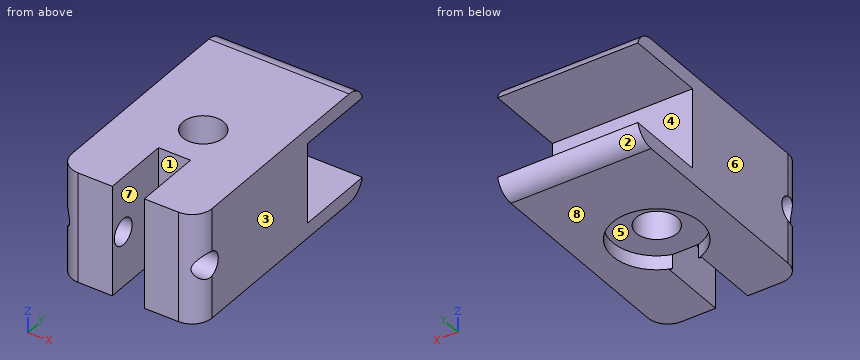
from build123d import *

# Parameters (mm, degrees)
CROQUIS1_W              = 35
CROQUIS1_H              = 35
CROQUIS1_R              = 11
ENTRADABASE_DEPTH       = 3.5
CROQUIS2_W              = 35
CROQUIS2_H              = 35
CROQUIS2_R              = 5.1
ENTRADACAVIDAD_DEPTH    = 24
REDONDEO1_R             = 5
CROQUIS4_W              = 27.5
CROQUIS4_H              = 14.86
CROQUIS4_R              = 3.25
BARRENORODAMIENTO_DEPTH = 35
CROQUIS5_W              = 8
CROQUIS5_H              = 16.86
ENTRADARODAMIENTO_DEPTH = 64.195487181
DETALLE2_R              = 5
CROQUIS10_W             = 3.75
CROQUIS10_H             = 15
SALIENTE_EXTRUIR4_DEPTH = 35
REDONDEO5_R             = 5
CROQUIS11_W             = 20
CROQUIS11_H             = 20
CORTAR_EXTRUIR5_DEPTH   = 64.195487351


with BuildPart() as part:
    # Croquis1 → EntradaBase (new body)
    with BuildSketch(Plane.XY):
        with Locations((17.5, -17.5)):
            Rectangle(CROQUIS1_W, CROQUIS1_H)
        with Locations((17.5, -17.5)):
            Circle(CROQUIS1_R, mode=Mode.SUBTRACT)
    extrude(amount=ENTRADABASE_DEPTH)

    # Croquis2 → EntradaCavidad (add)
    with BuildSketch(Plane.XY.offset(3.5)):
        with Locations((17.5, -17.5)):
            Rectangle(CROQUIS2_W, CROQUIS2_H)
        with Locations((17.5, -17.5)):
            Circle(CROQUIS2_R, mode=Mode.SUBTRACT)
    extrude(amount=ENTRADACAVIDAD_DEPTH)

    # Redondeo1
    redondeo1_edges = [part.edges().sort_by_distance(p)[0] for p in [
        (35, -35, 13.75),
        (0, -35, 13.75),
    ]]
    fillet(redondeo1_edges, radius=REDONDEO1_R)

    # Croquis4 → BarrenoRodamiento (add, through all)
    with BuildSketch(Plane.ZY):
        with Locations((13.75, -37.43)):
            Rectangle(CROQUIS4_W, CROQUIS4_H)
        with Locations(Location((13.75, -40.86, 0), (0, 0, 270))):
            Circle(CROQUIS4_R, mode=Mode.SUBTRACT)
    extrude(amount=-BARRENORODAMIENTO_DEPTH)

    # Croquis5 → EntradaRodamiento (cut, through all)
    with BuildSketch(Plane(origin=(0, 0, 0), x_dir=(-1, 0, 0), z_dir=(0, 0, -1))):
        with Locations((-17.5, -36.43)):
            Rectangle(CROQUIS5_W, CROQUIS5_H)
    extrude(amount=-ENTRADARODAMIENTO_DEPTH, mode=Mode.SUBTRACT)

    # Detalle2
    # the kernel refuses this fillet: 5 mm, written as the material it takes off along each edge
    with BuildSketch(Plane(origin=(35, -44.86, -12.5), x_dir=(-1, 0, 0), z_dir=(0, 0, 1))) as detalle2_piece_1:
        with BuildLine():
            CenterArc((DETALLE2_R, -DETALLE2_R), DETALLE2_R, 90, 90)
            Line((0, -DETALLE2_R), (0, 0))
            Line((0, 0), (DETALLE2_R, 0))
        make_face()
    extrude(amount=52.5, mode=Mode.SUBTRACT)
    with BuildSketch(Plane(origin=(0, -44.86, -12.5), x_dir=(1, 0, 0), z_dir=(0, 0, 1))) as detalle2_piece_2:
        with BuildLine():
            CenterArc((DETALLE2_R, DETALLE2_R), DETALLE2_R, 180, 90)
            Line((0, DETALLE2_R), (0, 0))
            Line((0, 0), (DETALLE2_R, 0))
        make_face()
    extrude(amount=52.5, mode=Mode.SUBTRACT)

    # Croquis10 → Saliente-Extruir4 (add, through all)
    with BuildSketch(Plane.ZY):
        with Locations((1.875, 7.5)):
            Rectangle(CROQUIS10_W, CROQUIS10_H)
        with Locations((25.625, 7.5)):
            Rectangle(CROQUIS10_W, CROQUIS10_H)
    extrude(amount=-SALIENTE_EXTRUIR4_DEPTH)

    # Redondeo5
    # the kernel refuses this fillet: 5 mm, written as the material it takes off along each edge
    with BuildSketch(Plane(origin=(-12.103072957, 15, 0), x_dir=(0, -1, 0), z_dir=(1, 0, 0))) as redondeo5_piece_1:
        with BuildLine():
            CenterArc((4.841229183, -5), REDONDEO5_R, 90, 75.522487814)
            Line((0, -3.75), (-0.096824584, -3.725))
            ThreePointArc((-0.096824584, -3.725), (-0.1, -1.875), (-0.1, 0))
            Line((-0.1, 0), (0, 0.1))
            Line((0, 0.1), (4.841229183, 0.1))
            Line((4.841229183, 0.1), (4.841229183, 0))
        make_face()
    extrude(amount=59.206145914, mode=Mode.SUBTRACT)
    with BuildSketch(Plane(origin=(-12.103072957, 15, 27.5), x_dir=(0, -1, 0), z_dir=(1, 0, 0))) as redondeo5_piece_2:
        with BuildLine():
            CenterArc((4.841229183, 5), REDONDEO5_R, 194.477512186, 75.522487814)
            Line((0, 3.75), (-0.096824584, 3.725))
            ThreePointArc((-0.096824584, 3.725), (-0.1, 1.875), (-0.1, 0))
            Line((-0.1, 0), (0, -0.1))
            Line((0, -0.1), (4.841229183, -0.1))
            Line((4.841229183, -0.1), (4.841229183, 0))
        make_face()
    extrude(amount=59.206145914, mode=Mode.SUBTRACT)

    # Croquis11 → Cortar-Extruir5 (cut, through all)
    with BuildSketch(Plane.ZY):
        with Locations((13.75, 5)):
            Rectangle(CROQUIS11_W, CROQUIS11_H)
    extrude(amount=-CORTAR_EXTRUIR5_DEPTH, mode=Mode.SUBTRACT)


solid = part.part
The listing builds one solid part. Answer for the finished solid, in the listing's coordinates (mm). Face numbers are marked on the shaded views. A direction names the side the tool comes from. Round coordinates to 2 decimals unless told otherwise and drop trailing zeros. Write each loop counter-clockwise with the first axis right and the second up, starting at its lowest first coordinate (ties: lowest second). Pieces come first, ordered by that corner, then holes. Notation, with made-up numbers: (54, 78) - (88, 78) arc R11 cw to (88, 92) - close; hole circle Ø9 at (77.25, 45). An arc over 180 degrees is marked (long way). Use a Markdown table: item, result. Add a question column.
1. The part is cut by section B-B (y = -32). Write down the section's boundary in (x, z), and give its area (4 significant figures).
2. A tool of negligible diameter and unlimited length cuts with its end or side. For the marked faces 1, 2, 3, 4 and 5, from which of +Z, -Z, +X, -X, +Y, -Y can it reach the whole face along a straight path? Write none if from no direction.
3. The part is cut by section A-A (x = 17.5). Write down the section's boundary in (y, z).
4. Consider line 1 (X direction, y = -32, z = 19.5); line 2 (Z direction, x = 13.5, y = -4); line 3 (Y direction, x = 25.5, z = 13.75). Determine where each line is inside the solid, lowest interval first.
5. For a pull along X with two mould halves and no side action, classify the marked faces 6, 7 and 8 as +X half, -X half, draft (parallel to the pull), parting line (faces both ways), or undercut.
6. The part is cut by section C-C (z = 15.5). Write down the section's boundary in (x, y).
7. The part is cut by section D-D (z = 4.5). Write down the section's boundary in (x, y), and give its area (3 significant figures).
8. Flat-ended cylindrical pins translate along their axes: P1, Ø1, axis at x = 20, z = 20, coming from the -Y side; P2, Ø10, axis at x = 20.5, z = 16.5, coming from the +Y side. Find the tip coordinate at first contact, or state that the pin passes through.
Reported:
| question | item | result |
|---|---|---|
| 1 | outline | (0, 0) - (13.5, 0) - (13.5, 27.5) - (0, 27.5) - close; (21.5, 0) - (35, 0) - (35, 27.5) - (21.5, 27.5) - close |
| 1 | area | 742.5 mm^2 |
| 2 | face 1 | +Z, -Z, -Y |
| 2 | face 2 | -Z, +X, -X, +Y |
| 2 | face 3 | +Z, -Z, +X, +Y, -Y |
| 2 | face 4 | +X, -X, +Y |
| 2 | face 5 | -Z |
| 3 | outline | (-28, 3.5) - (-22.6, 3.5) - (-22.6, 27.5) - (-28, 27.5) - close; (-12.4, 3.5) - (-6.5, 3.5) - (-6.5, 0) - (10.16, 0) arc R5 ccw to (15, 3.75) - (-5, 3.75) - (-5, 23.75) - (15, 23.75) arc R5 ccw to (10.16, 27.5) - (-12.4, 27.5) - close |
| 4 | line 1 | 0 to 13.5, 21.5 to 35 |
| 4 | line 2 | 0 to 3.75, 23.75 to 27.5 |
| 4 | line 3 | -44.86 to -44.11, -37.61 to -5 |
| 5 | face 6 | -X half |
| 5 | face 7 | undercut |
| 5 | face 8 | draft |
| 6 | outline | (0, -38.12) - (13.5, -38.12) - (13.5, -28) - (21.5, -28) - (21.5, -38.12) - (35, -38.12) - (35, -5) - (0, -5) - close; (1.68, -43.6) arc R5 ccw to (5, -44.86) - (13.5, -44.86) - (13.5, -43.6) - close; (21.5, -44.86) - (30, -44.86) arc R5 ccw to (33.32, -43.6) - (21.5, -43.6) - close; hole circle Ø10.2 at (17.5, -17.5) |
| 7 | outline | (0, -39.86) arc R5 ccw to (5, -44.86) - (13.5, -44.86) - (13.5, -28) - (21.5, -28) - (21.5, -44.86) - (30, -44.86) arc R5 ccw to (35, -39.86) - (35, -5) - (0, -5) - close; hole circle Ø10.2 at (17.5, -17.5) |
| 7 | area | 1,170 mm^2 |
| 8 | P1 | y = -28 |
| 8 | P2 | y = -5 |
